The listing builds one solid part. Answer for the finished solid, in the listing's coordinates (mm). Face numbers are marked on the shaded views. Round coordinates to 2 decimals unless told otherwise and drop trailing zeros. Order: outer loops, then holes, each group sorted by start corner. A loop starts at its lowest first (then second) coordinate and runs counter-clockwise, first axis right, second up. Notation, with made-up numbers: (61.25, -3.75) - (65.25, -3.75) arc R18 ccw to (65.25, 3.25) - close; hole circle Ø10 at (13.25, -35). An arc over 180 degrees is marked (long way). One line per item, written item: value. Start each with the question number.
1. Flat-ended cylindrical pins translate along their axes: P1, Ø10, axis at x = 13, y = 39, coming from the +Z side; P2, Ø1.5, axis at x = 10, y = 28.5, coming from the -Z side. Find the tip coordinate at first contact, or state that the pin passes through.
2. Straight lines are drawn through the part: line 1 (X direction, y = 49.5, z = 9.25); line 2 (Z direction, x = -6.5, y = 22); line 3 (Y direction, x = 22, z = 4). For each, find the intervals that lie inside material, in ascending order.
3. For a pull along Y with two mould halves and no side action, classify the marked faces 1, 2 and 3 as released by +Y, released by -Y, zero draft, split by the parting line, or undercut.
4. Section A-A, the plane y = 39.5 is taken. Give the vertices of the cut face in (x, z).
5. Section B-B, the plane x = -18 is taken. Give the vertices of the cut face in (y, z), then the cut area to 3 significant figures.
from build123d import *

# Parameters (mm, degrees)
F1_DEPTH = 7
F2_W     = 46.7807637383
F2_H     = 105.2663818344
F3_DEPTH = 2
F4_DEPTH = 3


with BuildPart() as f1:
    # F0 (on Top) → F1 (new body)
    with BuildSketch(Plane.XY):
        with BuildLine():
            Line((19.0969404806, 57.5190660946), (-27.6838232577, 57.5190660946))
            ThreePointArc((-27.6838232577, 57.5190660946), (-31.2193571636, 56.0546000006), (-32.6838232577, 52.5190660946))
            Line((-32.6838232577, 52.5190660946), (-32.6838232577, -52.7473157398))
            ThreePointArc((-32.6838232577, -52.7473157398), (-31.2193571636, -56.2828496457), (-27.6838232577, -57.7473157398))
            Line((-27.6838232577, -57.7473157398), (19.0969404806, -57.7473157398))
            ThreePointArc((19.0969404806, -57.7473157398), (22.6324743865, -56.2828496457), (24.0969404806, -52.7473157398))
            Line((24.0969404806, -52.7473157398), (24.0969404806, 52.5190660946))
            ThreePointArc((24.0969404806, 52.5190660946), (22.6324743865, 56.0546000006), (19.0969404806, 57.5190660946))
        make_face()
    extrude(amount=F1_DEPTH)

    # F2 (on face) → F3 (join)
    with BuildSketch(Plane.XY.offset(7)):
        with Locations((-4.2934413886, -0.1141248226)):
            Rectangle(F2_W, F2_H)
    extrude(amount=F3_DEPTH)

    # F4 (add): a face of the model
    f4_faces = [f1.faces().sort_by_distance(p)[0] for p in [
        (22.8120127039, -0.1141248226, 7),
    ]]
    extrude(f4_faces, amount=F4_DEPTH)


solid = f1.part
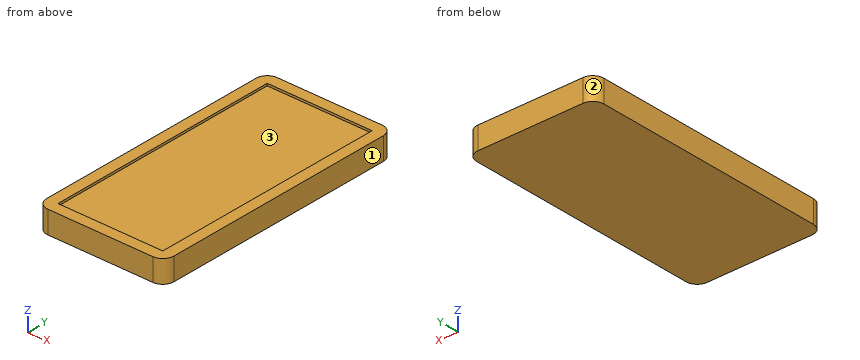
Answer list:
1. P1: stops at z = 9
1. P2: stops at z = 0
2. line 1: x = -32.68 to -27.68, 19.1 to 24.1
2. line 2: z = 0 to 9
2. line 3: y = -56.82 to 56.59
3. face 1: zero draft
3. face 2: released by +Y
3. face 3: undercut
4. outline: (-32.68, 0) - (24.1, 0) - (24.1, 10) - (19.1, 10) - (19.1, 9) - (-27.68, 9) - (-27.68, 10) - (-32.68, 10) - close
5. outline: (-57.75, 0) - (57.52, 0) - (57.52, 10) - (52.52, 10) - (52.52, 9) - (-52.75, 9) - (-52.75, 10) - (-57.75, 10) - close
5. area: 1,050 mm²
